Verification items for the finished model (mm, model axes). A direction names the side the tool comes from. Give positions to 0.01 mm unless a question says otherwise; leave off trailing zeros. Write each loop counter-clockwise with the first axis right and the second up, starting at its lowest first coordinate (ties: lowest second). Pieces come first, ordered by that corner, then holes. Notation, with made-up numbers: (29.25, 72) -> (51.25, 72) arc R29 ccw to (51.25, 102) -> close; hole circle Ø10 at (-34.5, 29.5). An arc over 180 degrees is marked (long way). Answer as CSV lines item,"result".
Autodesk Inventor part; units mm, degrees
ref_plane "YZ Plane" through (0, 0, 0) normal (1, 0, 0) x (0, 1, 0)
ref_plane "XZ Plane" through (0, 0, 0) normal (0, 1, 0) x (-1, 0, 0)
ref_plane "XY Plane" through (0, 0, 0) normal (0, 0, 1) x (1, 0, 0)
sketch "Skizze1" plane through (0, 0, 0) normal (1, 0, 0) x (0, 1, 0)
  circle A0 centre (0, 0) radius 75.5 construction
  arc A1 (-74.8348, 10) -> (-74.8348, -10) centre (0, 0) ccw
  line L0 (-74.8348, 10) -> (-69.5, 10)
  line L1 (-69.5, 10) -> (-69.5, -10)
  line L2 (-69.5, -10) -> (-74.8348, -10)
  point P0 (-75.5, 0)
  dimension "d3" = 151
  dimension "d4" = 6
  dimension "d5" = 20
extrude "Extrusion1" add sketch "Skizze1" along normal blind 25
sketch "Skizze2" plane through (0, -69.5, 10) normal (0, 1, 0) x (1, 0, 0)
  line L0 (0, 0) -> (5, 0)
  line L1 (5, 0) -> (5, 20)
  line L2 (5, 20) -> (0, 20)
  line L3 (0, 20) -> (0, 0)
  line L4 (0, 20) -> (25, 20)
  point P0 (0, 10)
  dimension "d8" = 5
extrude "Extrusion2" add sketch "Skizze2" along normal blind 20
sketch "Skizze3" plane through (25, -69.5, 10) normal (0, 1, 0) x (1, 0, 0)
  circle A0 centre (-10, 10) radius 3.25
  line L0 (-20, 20) -> (-20, 0) construction
  line L1 (-20, 0) -> (0, 0) construction
  line L2 (0, 20) -> (0, 0) construction
  line L3 (-20, 20) -> (0, 20) construction
  line L4 (-20, 20) -> (0, 0) construction
  line L5 (0, 20) -> (-20, 0) construction
  point P0 (-25, 10)
  dimension "d11" = 6.5
extrude "Extrusion4" cut sketch "Skizze3" against normal blind 10
properties part number "Slider_Winkel"
1) Scan lines: line 1 along Z through (x, y) = (15, -71.3); line 2 along X through (y, z) = (-70.85, 0); line 3 along X through (y, z) = (-58.25, 2.25). Record each from-to range of solid material in increasing order.
Reported:
line 1,"-10 to -3.25, 3.25 to 10"
line 2,"0 to 11.75, 18.25 to 25"
line 3,"0 to 5"
2) Section check D-D (y = -52.25). Record the boundary of the cut face in (x, z).
Reported:
outline,"(0, -10) -> (5, -10) -> (5, 10) -> (0, 10) -> close"
3) Section check B-B (x = 15). Record the boundary of the cut face in (y, z).
Reported:
outline,"(-75.43, -3.25) arc R75.5 ccw to (-74.83, -10) -> (-69.5, -10) -> (-69.5, -3.25) -> close; (-75.43, 3.25) -> (-69.5, 3.25) -> (-69.5, 10) -> (-74.83, 10) arc R75.5 ccw to start"
4) Depth check by flat-ended pin: pin 1 (6 mm diameter, centred on y = -62.5, z = 1, fed in from +X); pin 2 (5 mm diameter, centred on x = 4, z = -6.5, fed in from -Y). Enter the tip coordinate at first touch or a pass-through.
Reported:
pin 1,"x = 5"
pin 2,"y = -75.39"
5) Section check A-A (z = 0). Record the boundary of the cut face in (x, y).
Reported:
outline,"(0, -75.5) -> (11.75, -75.5) -> (11.75, -69.5) -> (5, -69.5) -> (5, -49.5) -> (0, -49.5) -> close; (18.25, -75.5) -> (25, -75.5) -> (25, -69.5) -> (18.25, -69.5) -> close"
6) Tool access check on faces 1 (the flat face through (5, -60, 0)), 2 (the flat face through (4, -68, -10)). Record the directions out of +Z, -Z, +X, -X, +Y, -Y that give a thin tool (end or side, any length) a straight path to the whole face; none if there is none.
Reported:
face 1,"+Z, -Z, +X, +Y"
face 2,"-Z, +X, -X, +Y, -Y"
7) Section check C-C (z = -3.75). Record the boundary of the cut face in (x, y).
Reported:
outline,"(0, -75.41) -> (25, -75.41) -> (25, -69.5) -> (5, -69.5) -> (5, -49.5) -> (0, -49.5) -> close"
